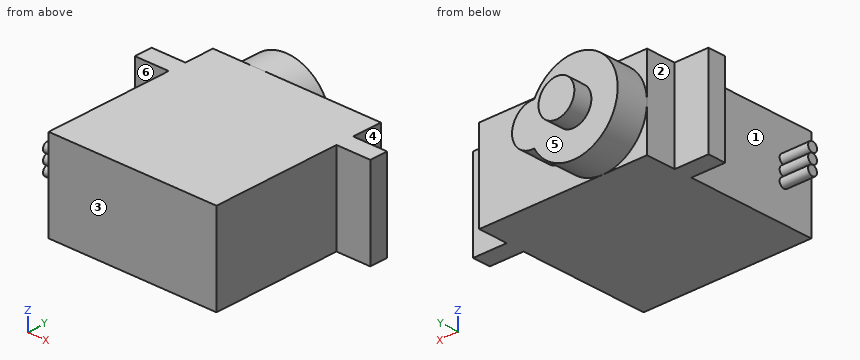
```python
from build123d import *

# Parameters (mm, degrees)
SKETCH1_W           = 22.95
SKETCH1_H           = 12.1
BOSS_EXTRUDE1_DEPTH = 24.1
BOSS_EXTRUDE2_DEPTH = 4.3
SKETCH3_W           = 4.625
SKETCH3_H           = 12.1
BOSS_EXTRUDE3_DEPTH = 2.45
SKETCH4_R           = 2.45
BOSS_EXTRUDE4_DEPTH = 2.5
SKETCH5_R           = 0.65
BOSS_EXTRUDE7_DEPTH = 3.9


with BuildPart() as part:
    # Sketch1 → Boss-Extrude1 (new body)
    with BuildSketch(Plane(origin=(0, 0, 0), x_dir=(1, 0, 0), z_dir=(0, 1, 0))):
        Rectangle(SKETCH1_W, SKETCH1_H)
    extrude(amount=BOSS_EXTRUDE1_DEPTH)

    # Sketch2 → Boss-Extrude2 (add)
    with BuildSketch(Plane(origin=(0, 24.1, 0), x_dir=(1, 0, 0), z_dir=(0, 1, 0))):
        with BuildLine():
            ThreePointArc((-0.056919643, 2.790378698), (-11.475, 0), (-0.056919643, -2.790378698))
            ThreePointArc((-0.056919643, -2.790378698), (2.975, 0), (-0.056919643, 2.790378698))
        make_face()
    extrude(amount=BOSS_EXTRUDE2_DEPTH)

    # Sketch3 → Boss-Extrude3 (add)
    with BuildSketch(Plane(origin=(0, 20.05, 0), x_dir=(1, 0, 0), z_dir=(0, 1, 0))):
        with Locations((-13.7875, 0)):
            Rectangle(SKETCH3_W, SKETCH3_H)
        with Locations((13.7875, 0)):
            Rectangle(SKETCH3_W, SKETCH3_H)
    extrude(amount=-BOSS_EXTRUDE3_DEPTH)

    # Sketch4 → Boss-Extrude4 (add)
    with BuildSketch(Plane(origin=(0, 28.4, 0), x_dir=(1, 0, 0), z_dir=(0, 1, 0))):
        with Locations((-5.425, 0)):
            Circle(SKETCH4_R)
    extrude(amount=BOSS_EXTRUDE4_DEPTH)

    # Sketch5 → Boss-Extrude7 (add)
    with BuildSketch(Plane.ZY.offset(11.475)):
        with Locations((0, 4)):
            Circle(SKETCH5_R)
        with Locations((1.34, 4)):
            Circle(SKETCH5_R)
        with Locations((-1.34, 4)):
            Circle(SKETCH5_R)
    extrude(amount=BOSS_EXTRUDE7_DEPTH)


solid = part.part
```
Geometry: final body of the model. Coordinates: model frame, mm. Face numbers are marked on the shaded views. A direction names the side the tool comes from. Round coordinates to 2 decimals unless told otherwise and drop trailing zeros. Write each loop counter-clockwise with the first axis right and the second up, starting at its lowest first coordinate (ties: lowest second). Pieces come first, ordered by that corner, then holes. Notation, with made-up numbers: M 53.5,-28.75 L 65.5,-28.75 A19 cw 65.5,7.25 Z; hole C 20.5,65 d8. An arc over 180 degrees is marked long. Answer in a Markdown table with one row per item. Add a question column.
(1) Cut plane D-D, the plane z = -4.25. Return the cut outline in (x, y) (3 decimals), then the cut area to 3 significant figures.
(2) Draft query along Y for the marked faces 1, 2 and 3. Return one class per face: pulls with the +Y half, pulls with the -Y half, needs draft (parallel to the pull), parting line crosses it, or undercut.
(3) Cut plane A-A, the plane z = -1.34. Return the cut outline in (x, y) (3 decimals), then the cut area to 3 significant figures.
(4) Ray query, L1, parallel to X at y = 12, z = -2.75 (3 decimals); L2, parallel to X at y = 29.5, z = 0 (3 decimals); L3, parallel to Y at x = 0, z = 1.75. Return the intervals inside material, ascending.
(5) Cut plane B-B, the plane x = -10. Return the cut outline in (y, z), then the cut area to 3 significant figures.
(6) Contact query for flat-ended pins moving along their axis: pin 1 (1.5 mm diameter, centred on y = 10, z = -2, fed in from +X) (3 decimals); pin 2 (5 mm diameter, centred on x = 10.5, z = -4, fed in from +Y); pin 3 (3.5 mm diameter, centred on x = 14, z = 1.5, fed in from +Y). Output: stop coordinate, or through.
(7) Cut plane C-C, the plane y = 8. Return the cut outline in (x, z) (3 decimals), then the cut area to 3 significant figures.
(8) Reachability of the marked faces 4, 5 and 6 from +Z, -Z, +X, -X, +Y, -Y: full face, straight path, thin tool, end or side. Return the list, or none.
Established:
| question | item | result |
|---|---|---|
| 1 | outline | M -16.1,17.6 L -11.475,17.6 L -11.475,0 L 11.475,0 L 11.475,17.6 L 16.1,17.6 L 16.1,20.05 L 11.475,20.05 L 11.475,24.1 L -1.119,24.1 L -1.119,28.4 L -9.731,28.4 L -9.731,24.1 L -11.475,24.1 L -11.475,20.05 L -16.1,20.05 Z |
| 1 | area | 613 mm² |
| 2 | face 1 | undercut |
| 2 | face 2 | needs draft |
| 2 | face 3 | pulls with the -Y half |
| 3 | outline | M -16.1,17.6 L -11.475,17.6 L -11.475,4.65 L -15.375,4.65 L -15.375,3.35 L -11.475,3.35 L -11.475,0 L 11.475,0 L 11.475,17.6 L 16.1,17.6 L 16.1,20.05 L 11.475,20.05 L 11.475,24.1 L 2.634,24.1 L 2.634,28.4 L -3.374,28.4 L -3.374,30.9 L -7.476,30.9 L -7.476,28.4 L -11.325,28.4 L -11.325,24.1 L -11.475,24.1 L -11.475,20.05 L -16.1,20.05 Z |
| 3 | area | 651 mm² |
| 4 | L1 | -11.475 to 11.475 |
| 4 | L2 | -7.875 to -2.975 |
| 4 | L3 | 0 to 28.4 |
| 5 | outline | M 0,-6.05 L 24.1,-6.05 L 24.1,-3.96 L 28.4,-3.96 L 28.4,3.96 L 24.1,3.96 L 24.1,6.05 L 0,6.05 Z |
| 5 | area | 326 mm² |
| 6 | pin 1 | x = 11.475 |
| 6 | pin 2 | y = 24.1 |
| 6 | pin 3 | y = 20.05 |
| 7 | outline | M -11.475,-6.05 L 11.475,-6.05 L 11.475,6.05 L -11.475,6.05 Z |
| 7 | area | 278 mm² |
| 8 | face 4 | +Z, -Z, +X, +Y |
| 8 | face 5 | +Y |
| 8 | face 6 | +Z, -Z, -X |
